Job drawing, mm, ordinate dimensions from the low corner. One solid piece. Coordinates: 2 decimals unless noted, no trailing zeros. Write each loop counter-clockwise with the first axis right and the second up, starting at its lowest first coordinate (ties: lowest second). Pieces come first, ordered by that corner, then holes. Notation, with made-up numbers: (-19, 22) -> (14, 22) arc R11 cw to (14, 31) -> close; hole circle Ø9 at (-39, 0). An arc over 180 degrees is marked (long way). Answer as a JSON object with one key per item and string values. Group by question number.
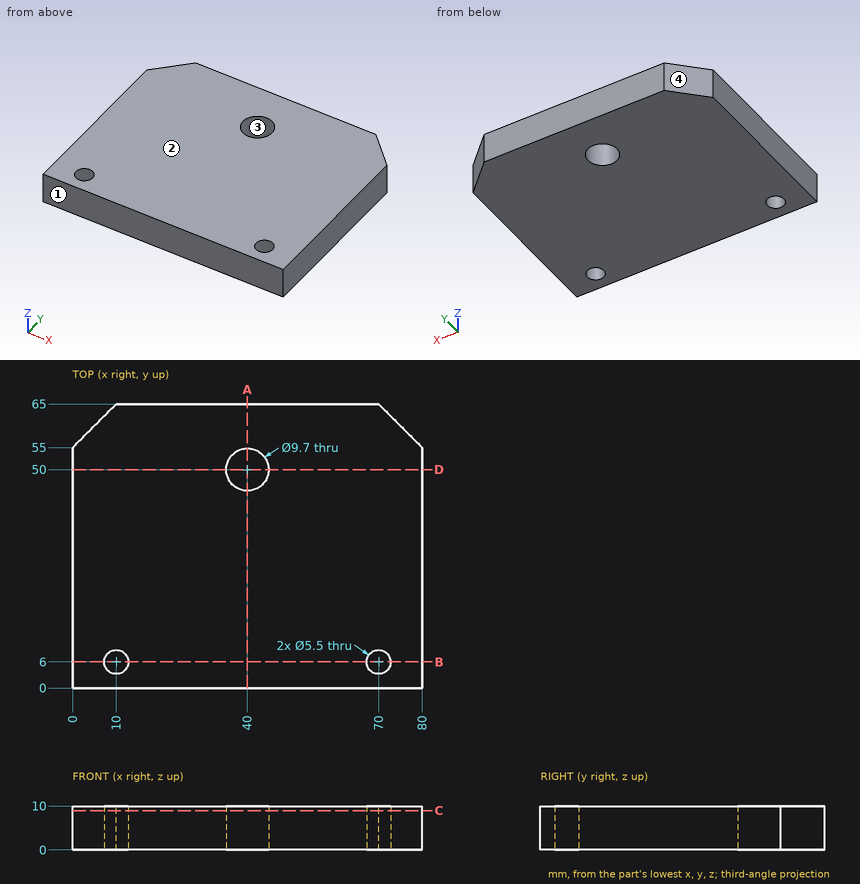
(1) Cut at C-C on z = 9. List the corners of the cut face in (x, y), plus the area to 3 significant figures.
(2) Pull direction Y, two halves, no side cores. Call the marked faces 1, 2, 3 and 4: released by +Y, released by -Y, zero draft, split by the parting line, or undercut.
(3) Pin check, flat tip, straight feed: pin 1 (3.5 mm diameter, centred on x = 10, y = 6, fed in from -Z). Stop position of the tip, or through.
(4) Cut at D-D on y = 50. List the corners of the cut face in (x, z), plus the area to 3 significant figures.
(5) Cut at B-B on y = 6. List the corners of the cut face in (x, z), plus the area to 3 significant figures.
(6) Cut at A-A on x = 40. List the corners of the cut face in (y, z), plus the area to 3 significant figures.
(7) Wall check: probe 1 along X at (y, z) = (6, 3); probe 2 along Y at (x, z) = (10, 5.5); probe 3 along X at (y, z) = (4.5, 1). Give the ranges that are in metal, low to high.
Results found:
{
 "1": {"outline": "(0, 0) -> (80, 0) -> (80, 55) -> (70, 65) -> (10, 65) -> (0, 55) -> close; hole circle Ø5.5 at (10, 6); hole circle Ø9.7 at (40, 50); hole circle Ø5.5 at (70, 6)", "area": "4,980 mm²"},
 "2": {"face 1": "released by -Y", "face 2": "zero draft", "face 3": "undercut", "face 4": "released by +Y"},
 "3": {"pin 1": "passes through"},
 "4": {"outline": "(0, 0) -> (35.15, 0) -> (35.15, 10) -> (0, 10) -> close; (44.85, 0) -> (80, 0) -> (80, 10) -> (44.85, 10) -> close", "area": "703 mm²"},
 "5": {"outline": "(0, 0) -> (7.25, 0) -> (7.25, 10) -> (0, 10) -> close; (12.75, 0) -> (67.25, 0) -> (67.25, 10) -> (12.75, 10) -> close; (72.75, 0) -> (80, 0) -> (80, 10) -> (72.75, 10) -> close", "area": "690 mm²"},
 "6": {"outline": "(0, 0) -> (45.15, 0) -> (45.15, 10) -> (0, 10) -> close; (54.85, 0) -> (65, 0) -> (65, 10) -> (54.85, 10) -> close", "area": "553 mm²"},
 "7": {"probe 1": "x = 0 to 7.25, 12.75 to 67.25, 72.75 to 80", "probe 2": "y = 0 to 3.25, 8.75 to 65", "probe 3": "x = 0 to 7.7, 12.3 to 67.7, 72.3 to 80"}
}
